Design review of the part shown in the three views and the two pictorial views. Dimensions are in mm from the part's minimum x, y and z. Coordinates: 2 decimals unless noted, no trailing zeros. Write item = value, one per line. Start each with the question number.
1) Consider section A-A on z = 47.5. State how many separate pieces and enclosed holes the cut face has, and give its area (3 significant figures).
2) Insertion check: pin 1 Ø3 at (x, z) = (2.5, 2.5) entering from +Y. The pin has a flat end and moves straight along its axis. Give the tip position at first contact, or say it passes through.
3) Wall thickness on probe 1 along X at (y, z) = (1.25, 3.5); probe 2 along Z at (x, y) = (67, 4.45): over which ranges is each line inside the solid? List them lowest first. Write a range as [from, to].
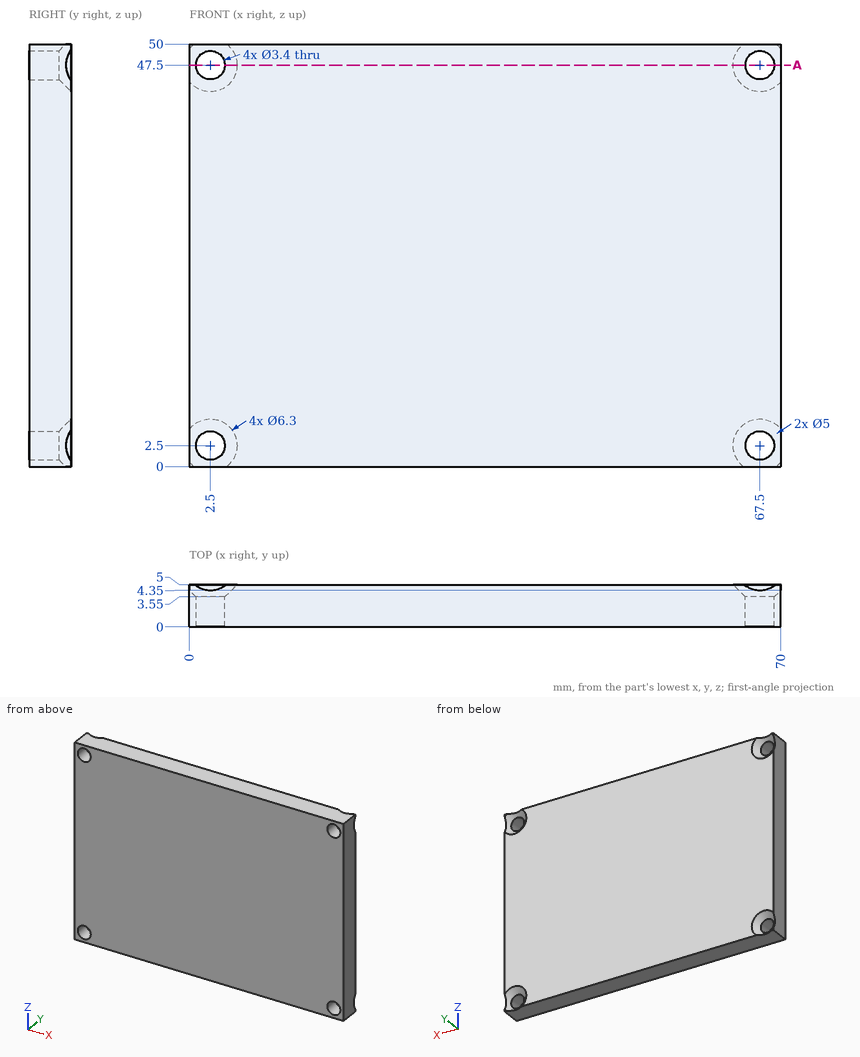
Answer sheet:
q1.separate_pieces = 3
q1.enclosed_holes = 0
q1.area = 312 mm2
q2.pin_1 = through
q3.probe_1 = [0, 1.13], [3.87, 66.13], [68.87, 70]
q3.probe_2 = [5.05, 44.95]
